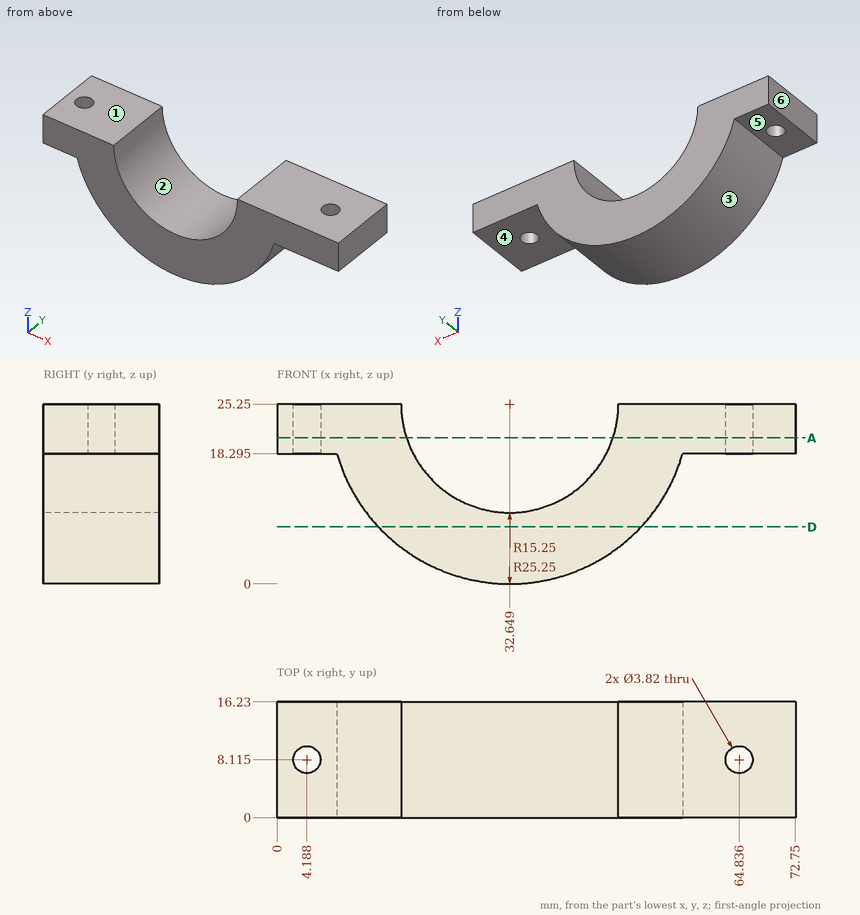
Geometry: see drawing. Coordinates: mm, zero at the bounding-box minimum. A direction names the side the tool comes from. Coordinates: 2 decimals unless noted, no trailing zeros. Write each loop counter-clockwise with the first axis right and the second up, starting at its lowest first coordinate (ties: lowest second). Pieces come first, ordered by that corner, then holes. Notation, with made-up numbers: M 58,-23.5 L 82,-23.5 A19 cw 82,-16.5 Z; hole C 14,46.5 d8. An arc over 180 degrees is marked long. Answer as a JSON object with one key per item and string values.
1. Draft query along X for the marked faces 1, 2 and 3. Return one class per face: released by +X, released by -X, zero draft, split by the parting line, or undercut.
Evaluation:
{"face 1": "zero draft", "face 2": "undercut", "face 3": "split by the parting line"}
2. Access query for the marked faces 4, 5 and 6. Directions: +Z, -Z, +X, -X, +Y, -Y. A direction counts if a zero-diameter tool reaches every point of the face in a straight line with its end or side. Return the directions, or none.
Evaluation:
{"face 4": "-Z, +X, +Y, -Y", "face 5": "-Z, -X, +Y, -Y", "face 6": "+Z, -Z, -X, +Y, -Y"}
3. Contact query for flat-ended pins moving along their axis: P1, Ø8, axis at x = 16.5, z = 15.5, coming from the -Y side; P2, Ø4, axis at y = 10, z = 11.5, coming from the +X side; P3, Ø2.5, axis at x = 64.84, y = 8.11, coming from the +Z side; P4, Ø2, axis at x = 29, y = 13, coming from the +Z side (1 decimal). Output: stop coordinate, or through.
Evaluation:
{"P1": "y = 0", "P2": "x = 55", "P3": "through", "P4": "z = 10.7"}
4. Ray query, L1, parallel to X at y = 13.5, z = 19; L2, parallel to Z at x = 32.5, y = 15.75; L3, parallel to Z at x = 44, y = 9.75 (1 decimal). Return the intervals inside material, ascending.
Evaluation:
{"L1": "0 to 18.74, 46.56 to 72.75", "L2": "0 to 10", "L3": "2.7 to 15.1"}
5. Cut plane D-D on z = 8. Output: boundary loops of the cut face in (x, y).
Evaluation:
{"outline": "M 14.21,0 L 51.09,0 L 51.09,16.23 L 14.21,16.23 Z"}
6. Cut plane A-A on z = 20.5. State how many separate pieces and enclosed holes the cut face has.
Evaluation:
{"separate pieces": "2", "enclosed holes": "2"}
